Source: CAD feature listing. Evaluate the final solid. Frame: model axes, mm. Coordinates: 2 decimals unless noted, no trailing zeros. Order: outer loops, then holes, each group sorted by start corner. A loop starts at its lowest first (then second) coordinate and runs counter-clockwise, first axis right, second up.
Item 1: Section C-C on z = 4.25. Return the cut outline in (x, y).
Item 2: Section A-A on x = 0. Return the cut outline in (y, z), then the cut area to 3 significant figures.
Item 3: Section D-D on x = 38. Return the cut outline in (y, z), then the cut area to 3 significant figures.
Item 4: Ray query, line 1 (Y direction, x = 0, z = 11.75); line 2 (X direction, y = -2.5, z = 2.75); line 3 (X direction, y = 11, z = 8). Return the intervals inside material, ascending.
Item 5: Mould query, pull axis X, two halves, no side actions, for faces 1 (the cylindrical face through (11.923, 3.755, 12.675)), 2 (the flat face through (10, -10, 0)), 3 (the cylindrical face through (-37.2, -28.5, 12.7)). Classes: released by +X, released by -X, zero draft, split by the parting line, or undercut.
Item 6: Contact query for flat-ended pins moving along their axis: P1, Ø6, axis at y = 35.5, z = 7, coming from the -X side; P2, Ø3, axis at x = -4, z = 18.5, coming from the +Y side; P3, Ø1, axis at x = -28, z = 3, coming from the -Y side. Output: stop coordinate, or through.
Autodesk Inventor part; units mm, degrees
ref_plane "YZ Plane" through (0, 0, 0) normal (1, 0, 0) x (0, 1, 0)
ref_plane "XZ Plane" through (0, 0, 0) normal (0, 1, 0) x (-1, 0, 0)
ref_plane "XY Plane" through (0, 0, 0) normal (0, 0, 1) x (1, 0, 0)
sketch "Sketch1" plane through (0, 0, 0) normal (0, 0, 1) x (1, 0, 0)
  circle A0 centre (0, 0) radius 75
  dimension "d0" = 150
extrude "Extrusion1" add sketch "Sketch1" along normal blind 25
fillet "Fillet1" radius 10 2 edges at (-75, 0, 25) (-75, 0, 0)
sketch "Sketch2" plane through (0, 0, 25) normal (0, 0, 1) x (1, 0, 0)
  circle A0 centre (0, 0) radius 12.5
  dimension "d4" = 25
extrude "Extrusion2" cut sketch "Sketch2" against normal blind 25
sketch "Sketch3" plane through (0, 0, 25) normal (0, 0, 1) x (1, 0, 0)
  point P0 (0, 0)
sketch "Sketch4" plane through (0, 0, 25) normal (0, 0, 1) x (1, 0, 0)
  circle A0 centre (0, 0) radius 46.8628
extrude "Extrusion3" cut sketch "Sketch4" against normal blind 25 keep common part
sketch "Sketch5" plane through (0, 0, 0) normal (0, 0, -1) x (-1, 0, 0)
  point P0 (0, 0)
sketch "Sketch6" plane through (0, 0, 25) normal (0, 0, 1) x (1, 0, 0)
  point P0 (0, 0)
properties part number "roller"
Answer list:
1. outline: circle Ø93.73 at (0, 0); hole circle Ø25 at (0, 0)
2. outline: (-46.86, 0) - (-12.5, 0) - (-12.5, 25) - (-46.86, 25) - close; (12.5, 0) - (46.86, 0) - (46.86, 25) - (12.5, 25) - close
2. area: 1,720 mm2
3. outline: (-27.42, 0) - (27.42, 0) - (27.42, 25) - (-27.42, 25) - close
3. area: 1,370 mm2
4. line 1: y = -46.86 to -12.5, 12.5 to 46.86
4. line 2: x = -46.8 to -12.25, 12.25 to 46.8
4. line 3: x = -45.55 to -5.94, 5.94 to 45.55
5. face 1: undercut
5. face 2: zero draft
5. face 3: split by the parting line
6. P1: stops at x = -33.76
6. P2: stops at y = 46.8
6. P3: stops at y = -37.95
